Build history of the part. All positions in model axes, mm. Face numbers are marked on the shaded views. A direction names the side the tool comes from. Coordinates: 2 decimals unless noted, no trailing zeros. Order: outer loops, then holes, each group sorted by start corner. A loop starts at its lowest first (then second) coordinate and runs counter-clockwise, first axis right, second up. Notation, with made-up numbers: (60, 61.5) - (106, 61.5) arc R19 cw to (106, 76.5) - close; hole circle Ø4 at (56, -1). An arc over 180 degrees is marked (long way). Write each question's results on one line, items separated by ' | '.
from build123d import *

# Parameters (mm, degrees)
WYCI_GNI_CIE_PO_CIE_CE_CIENKA_CIAN_2_R   = 10
WYCI_GNI_CIE_PO_CIE_CE_CIENKA_CIAN_2_R_2 = 7.5


with BuildPart() as part:
    # Wyci_gni_cie po _cie_ce-Cienka _cianka1: sweep along a curve in space
    with BuildLine() as wyci_gni_cie_po_cie_ce_cienka_cianka1_path:
        Line((344.842449098, -107.760635274, -45.933666989), (344.842449098, -107.760635274, -30.175831262))
        Line((344.842449098, -107.760635274, -30.175831262), (344.842449098, -107.760635274, -20.751368547))
        ThreePointArc((344.842449098, -107.760635274, -20.751368547), (344.842449098, -101.902770898, -6.609232923), (344.842449098, -87.760635274, -0.751368547))
        Line((344.842449098, -87.760635274, -0.751368547), (344.842449098, -84.035691476, -0.751368547))
        ThreePointArc((334.225321639, -66.373238459, -0.72656527), (341.983881451, -73.731732804, -0.744690484), (344.842449098, -84.035691476, -0.751368547))
        Line((334.225321639, -66.373238459, -0.72656527), (316.94225441, -57.191911349, -0.686189311))
        ThreePointArc((316.94225441, -57.191911349, -0.686189311), (258.162073815, -32.716996153, -0.548869578), (195.849321408, -19.630756919, -0.403297204))
        Line((195.849321408, -19.630756919, -0.403297204), (23.216575519, 0, 0))
        Line((23.216575519, 0, 0), (0, 0, 0))
    # Wyci_gni_cie po _cie_ce-Cienka _cian 2 (on start of the path) → Wyci_gni_cie po _cie_ce-Cienka _cianka1 (sweep)
    with BuildSketch(Plane(origin=(344.842449098, -107.760635274, -45.933666989), x_dir=(0, 1, 0), z_dir=(0, 0, 1))):
        Circle(WYCI_GNI_CIE_PO_CIE_CE_CIENKA_CIAN_2_R)
        Circle(WYCI_GNI_CIE_PO_CIE_CE_CIENKA_CIAN_2_R_2, mode=Mode.SUBTRACT)
    sweep(path=wyci_gni_cie_po_cie_ce_cienka_cianka1_path.line, transition=Transition.RIGHT)


solid = part.part
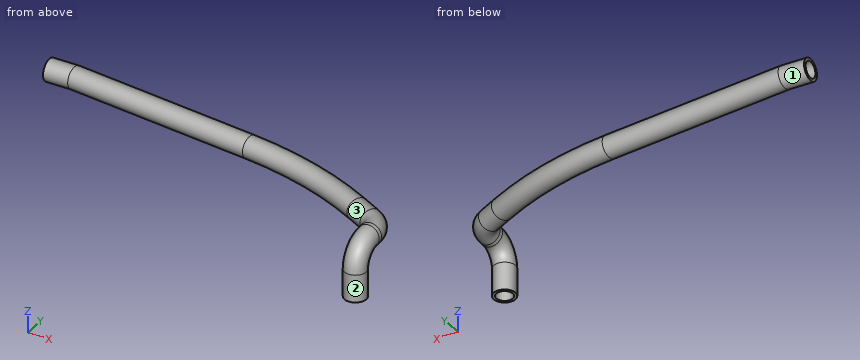
1. Drop flat-ended pins along their axis: pin 1 Ø6 at (x, y) = (89, -5.5) entering from +Z; pin 2 Ø6 at (x, z) = (205.5, 1) entering from +Y; pin 3 Ø12 at (x, z) = (344.84, -0.75) entering from -Y. Give the stop position or say it passes through.
Solved:
pin 1: stops at z = 9.85 | pin 2: stops at y = -10.4 | pin 3: stops at y = -114.29
2. Tool access for the marked faces 1, 2 and 3: list every direction of +Z, -Z, +X, -X, +Y, -Y with a clear straight run to the whole face (end or side of a thin tool).
Solved:
face 1: -X | face 2: -Z | face 3: none
3. Band-saw the part on A-A on z = -35. Give the cut face in (x, y).
Solved:
outline: circle Ø20 at (344.84, -107.76); hole circle Ø15 at (344.84, -107.76)
4. Probe line 1 (Z direction, x = 9.5, y = 0); line 2 (X direction, y = -75, z = -1). List the from-to ranges inside material, lowest first.
Solved:
line 1: z = -10 to -7.5, 7.5 to 10 | line 2: x = 329.16 to 333.49, 350.81 to 353.45
